Design review of the part shown in the three views and the two pictorial views. Dimensions are in mm from the part's minimum x, y and z. A direction names the side the tool comes from. Coordinates: 2 decimals unless noted, no trailing zeros. Loops run counter-clockwise (first coordinate to the right, second up) from the corner with the lowest first, then second, coordinate; pieces in that order, holes last. Notation, with made-up numbers: (-23, 71.25) -> (-19, 71.25) arc R35 cw to (-19, 105.25) -> close; hole circle Ø7 at (51, 18.5). An arc over 180 degrees is marked (long way). One line per item, written item: value. Start each with the question number.
1. Machinability: for the marked faces 4, 5, 6 and 7, which of the approach directions +Z, -Z, +X, -X, +Y, -Y give a long, thin tool a straight path to every point of the face, cutting with its end or side? Answer none if there is none.
2. Draft analysis for pull direction Z (two halves, no side actions). For the marked faces 1, 2 and 3, state which applies: pulls with the +Z half, pulls with the -Z half, needs draft (parallel to the pull), parting line crosses it, or undercut.
3. Add section B-B on z = 6. Write out the cut boundary in (x, y), plus the area to 3 significant figures.
4. Add section D-D on y = 6.5. Write out the cut boundary in (x, z).
5. Add section A-A on y = 22.5. Write out the cut boundary in (x, z).
6. For probe 1 along X at (y, z) = (3, 46); probe 2 along Z at (x, y) = (28, 2.55); probe 3 along X at (y, z) = (30.5, 32), list the stretches that pass through material, from the lowest coordinate up.
7. Add section C-C on x = 9. Write out the cut boundary in (y, z).
8. Insertion check: pin 1 (3.5 mm diameter, centred on x = 1.5, z = 28, fed in from -Y); pin 2 (14 mm diameter, centred on x = 18, y = 23.5, fed in from +Z); pin 3 (0.9 mm diameter, centred on x = 1.5, y = 2, fed in from +Z). Each pin has a flat end and moves straight along its axis. Give the tip position at first contact, or say it passes through.
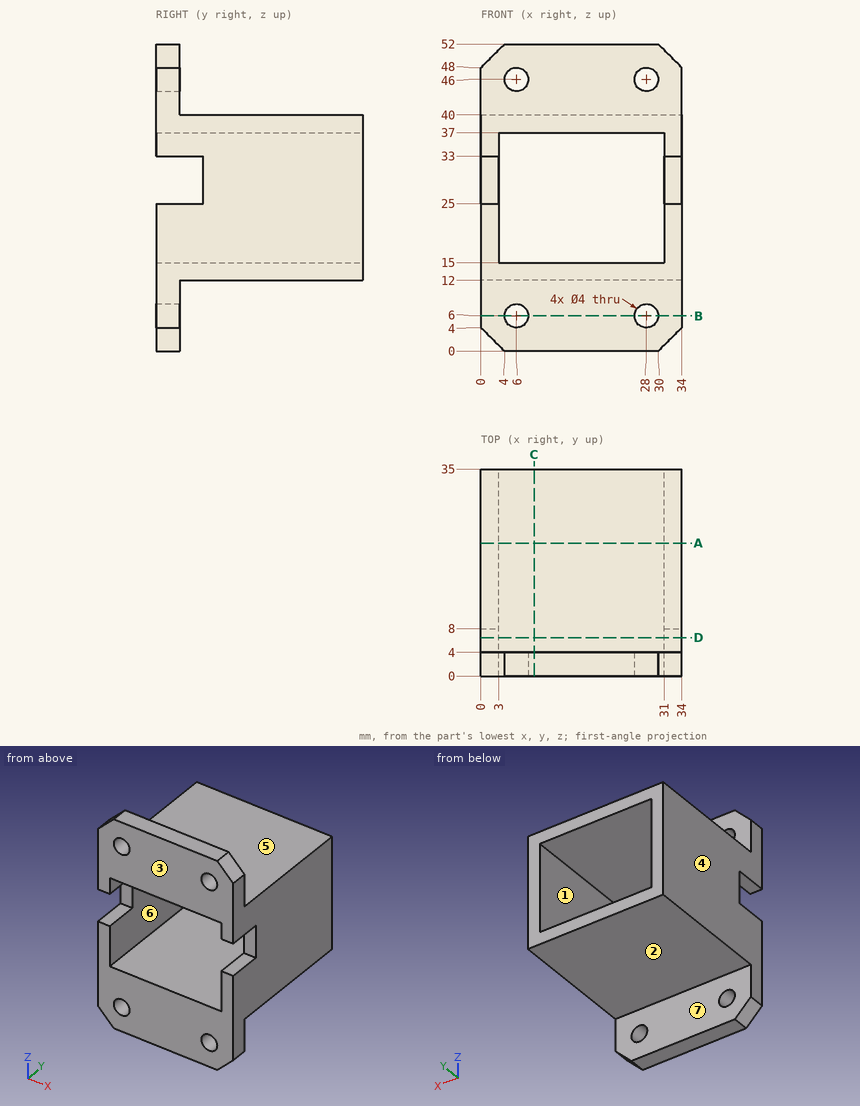
Worked answers:
1. face 4: +Z, -Z, -X, +Y, -Y
1. face 5: +Z, +X, -X, +Y
1. face 6: +Y, -Y
1. face 7: -Z, +X, -X, +Y
2. face 1: undercut
2. face 2: pulls with the -Z half
2. face 3: needs draft
3. outline: (0, 0) -> (4, 0) -> (4, 4) -> (0, 4) -> close; (8, 0) -> (26, 0) -> (26, 4) -> (8, 4) -> close; (30, 0) -> (34, 0) -> (34, 4) -> (30, 4) -> close
3. area: 104 mm²
4. outline: (0, 12) -> (34, 12) -> (34, 25) -> (31, 25) -> (31, 15) -> (3, 15) -> (3, 25) -> (0, 25) -> close; (0, 33) -> (3, 33) -> (3, 37) -> (31, 37) -> (31, 33) -> (34, 33) -> (34, 40) -> (0, 40) -> close
5. outline: (0, 12) -> (34, 12) -> (34, 40) -> (0, 40) -> close; hole (3, 15) -> (31, 15) -> (31, 37) -> (3, 37) -> close
6. probe 1: x = 0 to 4, 8 to 26, 30 to 34
6. probe 2: z = 0 to 4, 8 to 15, 37 to 44, 48 to 52
6. probe 3: x = 0 to 3, 31 to 34
7. outline: (0, 0) -> (4, 0) -> (4, 12) -> (35, 12) -> (35, 15) -> (0, 15) -> close; (0, 37) -> (35, 37) -> (35, 40) -> (4, 40) -> (4, 52) -> (0, 52) -> close
8. pin 1: stops at y = 8
8. pin 2: stops at z = 40
8. pin 3: stops at z = 49.95
